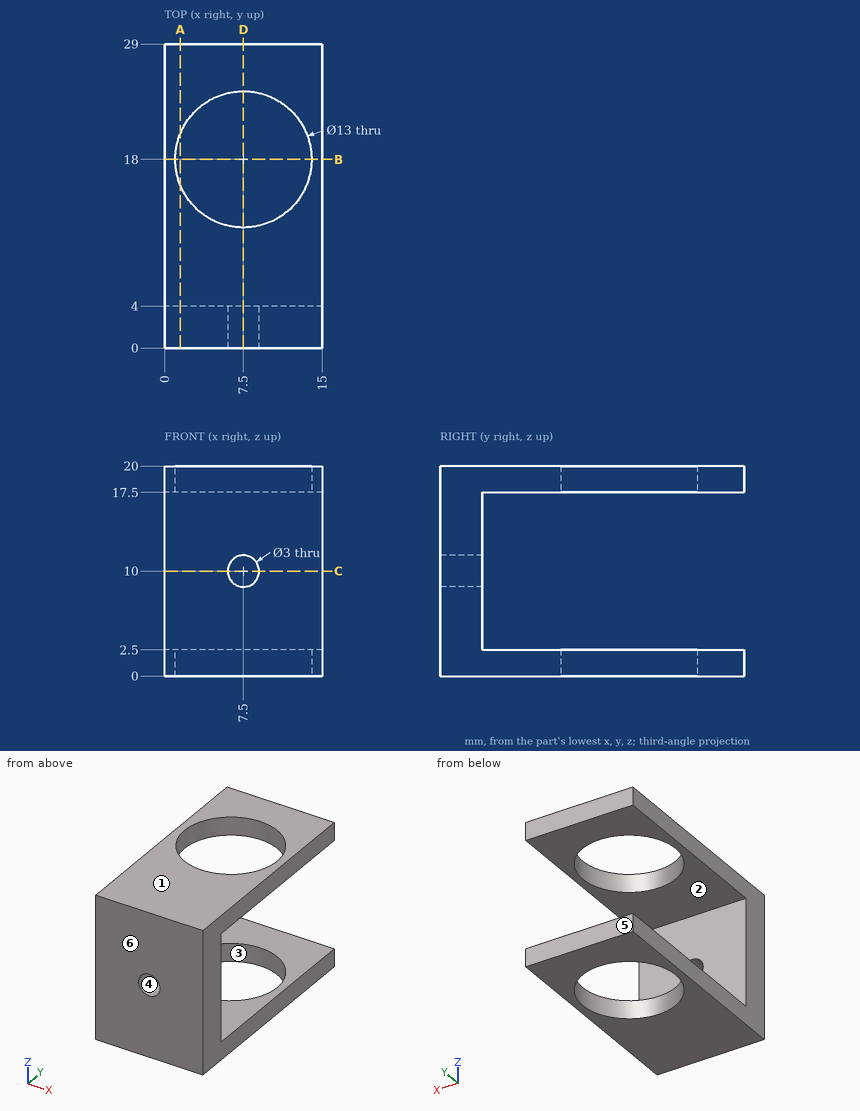
For this review, use the dimensioned drawing (mm, ordinates from the lowest corner) and the shaded views. A direction names the side the tool comes from. Round coordinates to 2 decimals unless told otherwise and drop trailing zeros. Write each loop counter-clockwise with the first axis right and the second up, starting at its lowest first coordinate (ties: lowest second). Pieces come first, ordered by that corner, then holes. Notation, with made-up numbers: M -37.75,-39.5 L -30.75,-39.5 A8 ccw -30.75,-32.5 Z; hole C -10,56 d3. An arc over 180 degrees is marked long. Answer as CSV lines item,"result". Start each with the question number.
Q1. Tool access review of the marked faces 1 and 2: name each direction out of +Z, -Z, +X, -X, +Y, -Y from which nothing blocks a thin tool from reaching the whole face with its end or side.
Q2. Consider section C-C, the plane z = 10. Give the boundary of the cut face in (x, y).
Q3. Wall thickness on line 1 along Z through (x, y) = (6.25, 5.25); line 2 along Z through (x, y) = (7.5, 1.6); line 3 along Y through (x, z) = (7.5, 18.1): over which ranges is each line inside the solid? List them lowest first.
Q4. Consider section A-A, the plane x = 1.5. Give the boundary of the cut face in (y, z), then the cut area to 3 significant figures.
Q5. Clearance check with flat-ended pins moving along their axes: P1, Ø8, axis at x = 8.5, y = 3.5, coming from the -Z side; P2, Ø4.5, axis at x = 11, y = 16, coming from the -Z side. State where each tip first meets the part, or that it passes through.
Q6. The part is to be moulded in two halves that separate along Y. For the marked faces 3, 4, 5 and 6, say which applies: +Y half, -Y half, draft (parallel to the pull), parting line (faces both ways), or undercut.
Q7. Consider section B-B, the plane y = 18. Give the boundary of the cut face in (x, z).
Q8. Consider section D-D, the plane x = 7.5. Give the boundary of the cut face in (y, z).
Result set:
1,face 1,"+Z, +X, -X, +Y, -Y"
1,face 2,"+X, -X, +Y"
2,outline,"M 0,0 L 6,0 L 6,4 L 0,4 Z; M 9,0 L 15,0 L 15,4 L 9,4 Z"
3,line 1,"z = 0 to 2.5, 17.5 to 20"
3,line 2,"z = 0 to 8.5, 11.5 to 20"
3,line 3,"y = 0 to 11.5, 24.5 to 29"
4,outline,"M 0,0 L 15.5,0 L 15.5,2.5 L 4,2.5 L 4,17.5 L 15.5,17.5 L 15.5,20 L 0,20 Z; M 20.5,0 L 29,0 L 29,2.5 L 20.5,2.5 Z; M 20.5,17.5 L 29,17.5 L 29,20 L 20.5,20 Z"
4,area,"180 mm²"
5,P1,"stops at z = 0"
5,P2,"passes through"
6,face 3,"undercut"
6,face 4,"draft"
6,face 5,"+Y half"
6,face 6,"-Y half"
7,outline,"M 0,0 L 1,0 L 1,2.5 L 0,2.5 Z; M 0,17.5 L 1,17.5 L 1,20 L 0,20 Z; M 14,0 L 15,0 L 15,2.5 L 14,2.5 Z; M 14,17.5 L 15,17.5 L 15,20 L 14,20 Z"
8,outline,"M 0,0 L 11.5,0 L 11.5,2.5 L 4,2.5 L 4,8.5 L 0,8.5 Z; M 0,11.5 L 4,11.5 L 4,17.5 L 11.5,17.5 L 11.5,20 L 0,20 Z; M 24.5,0 L 29,0 L 29,2.5 L 24.5,2.5 Z; M 24.5,17.5 L 29,17.5 L 29,20 L 24.5,20 Z"
